Here's how the part is built. I have some questions about the finished solid (model axes, mm). Face numbers are marked on the shaded views. A direction names the side the tool comes from. Coordinates: 2 decimals unless noted, no trailing zeros. Write each loop counter-clockwise with the first axis right and the second up, starting at its lowest first coordinate (ties: lowest second). Pieces come first, ordered by that corner, then holes. Notation, with made-up numbers: (-27.5, -7.75) -> (11.5, -7.75) arc R34 cw to (11.5, 23.25) -> close; hole circle Ø3 at (43, 68.5). An arc over 180 degrees is marked (long way). Put each result on its own line as item: value. Start each with the question number.
Item 1: If we mould it in two halves opening along Y, with no side actions, what happens to the marked faces 1, 2 and 3? For each: released by +Y, released by -Y, zero draft, split by the parting line, or undercut.
Item 2: I want a section at A-A, the plane y = -4. List the corners of the cut face in (x, z) for me.
Item 3: I want a section at C-C, the plane x = -16. List the corners of the cut face in (y, z) for me.
Item 4: For pin 1 (5 mm diameter, centred on y = 0.5, z = 6, fed in from -X); pin 2 (5 mm diameter, centred on x = -6, z = 3, fed in from +Y); pin 3 (1.5 mm diameter, centred on x = -14.5, z = 7, fed in from +Y); pin 4 (1 mm diameter, centred on x = 14, y = 2.5, fed in from -Z), each with a flat end and sliding along its axis, tell me the tip position at first contact or that it passes through.
Item 5: I need wall thicknesses on line 1 (Y direction, x = 0, z = 4); line 2 (X direction, y = -4, z = 6.5); line 3 (X direction, y = 24, z = 6.5). Which ranges of each line are inside material? Lowest first, please. Write a range as [from, to].
Item 6: On a 3-axis mill with a long thin cutter (end or side, diameter ignored), from which of +Z, -Z, +X, -X, +Y, -Y can I reach the whole of each face in a straight line? I mean the marked faces 4, 5, 6 and 7. Say none if no direction works.
Item 7: I want a section at B-B, the plane x = 0. List the corners of the cut face in (y, z) for me.
from build123d import *

# Parameters (mm, degrees)
F0_W     = 2
F0_H     = 4
F0_H_2   = 2.8740456328
F1_DEPTH = 10
F2_R     = 0.99999


# Not quite as in the source:
# - a fillet or chamfer is up to 0.001 mm smaller than in the source, because OpenCascade refuses the exact size


with BuildPart() as f1:
    # F0 (on Top) → F1 (new body)
    with BuildSketch(Plane.XY):
        Polygon((14.5, 18.75), (-14.5, 18.75), (-14.5, 13.8759543672), (-14.5, 9.8759543672), (-14.5, -18.75), (14.5, -18.75), (14.5, 9.8759543672), (14.5, 13.8759543672), align=None)
        Polygon((-13, 4.7144976147), (-13, 17.25), (13, 17.25), (13, 4.7144976147), (13, -2.2855023853), (13, -17.25), (-13, -17.25), (-13, -2.2855023853), align=None, mode=Mode.SUBTRACT)
        with Locations((-15.5, 11.8759543672)):
            Rectangle(F0_W, F0_H)
        Polygon((-16.5, 9.8759543672), (-16.5, 13.8759543672), (-16.5, 29.8609879265), (-19.8, 24.85), (-18, 24.85), (-18, 12.75), (-18, 9.8759543672), align=None)
        with Locations((15.5, 11.8759543672)):
            Rectangle(F0_W, F0_H)
        Polygon((16.5, 29.8609879265), (16.5, 13.8759543672), (16.5, 9.8759543672), (18, 9.8759543672), (18, 12.75), (18, 24.85), (19.8, 24.85), align=None)
        with Locations((-19, 11.3129771836)):
            Rectangle(F0_W, F0_H_2)
        with Locations((19, 11.3129771836)):
            Rectangle(F0_W, F0_H_2)
    extrude(amount=F1_DEPTH)

    # F2 (radius 1 in the source; OpenCascade refuses exactly that, so slightly less here)
    f2_edges = [f1.edges().sort_by_distance(p)[0] for p in [
        (-14.5, 18.75, 5),
        (-20, 9.875954, 5),
        (14.5, 18.75, 5),
        (20, 9.875954, 5),
        (-13, 17.25, 5),
        (14.5, 9.875954, 5),
        (14.5, -18.75, 5),
        (-14.5, -18.75, 5),
        (-13, -17.25, 5),
        (13, 17.25, 5),
        (13, -17.25, 5),
        (-14.5, 13.875954, 5),
        (16.5, 13.875954, 5),
        (-16.5, 13.875954, 5),
        (14.5, 13.875954, 5),
        (-16.5, 29.860988, 5),
        (16.5, 29.860988, 5),
    ]]
    fillet(f2_edges, radius=F2_R)


solid = f1.part
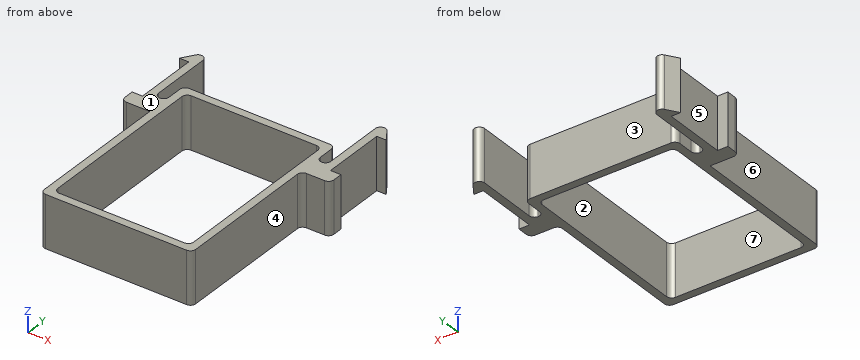
Calculated:
1. face 1: zero draft
1. face 2: undercut
1. face 3: released by +Y
2. outline: (-14.5, 0) -> (-13, 0) -> (-13, 10) -> (-14.5, 10) -> close; (13, 0) -> (14.5, 0) -> (14.5, 10) -> (13, 10) -> close
3. outline: (9.88, 0) -> (14.01, 0) -> (14.01, 10) -> (9.88, 10) -> close
4. pin 1: stops at x = -14.5
4. pin 2: stops at y = 18.75
4. pin 3: stops at y = 18.72
4. pin 4: stops at z = 0
5. line 1: y = [-18.75, -17.25], [17.25, 18.75]
5. line 2: x = [-14.5, -13], [13, 14.5]
5. line 3: x = [-18, -16.5], [16.5, 18]
6. face 4: +Z, -Z, +X, -Y
6. face 5: +Z, -Z, -X
6. face 6: +Z, -Z, -X, -Y
6. face 7: +Z, -Z
7. outline: (-18.75, 0) -> (-17.25, 0) -> (-17.25, 10) -> (-18.75, 10) -> close; (17.25, 0) -> (18.75, 0) -> (18.75, 10) -> (17.25, 10) -> close
